The figure shows three views and two pictorial views of one solid part (mm, origin at its lowest corner). Answer the questions. A direction names the side the tool comes from. Coordinates: 2 decimals unless noted, no trailing zeros. Write each loop counter-clockwise with the first axis right and the second up, starting at its lowest first coordinate (ties: lowest second). Pieces come first, ordered by that corner, then holes.
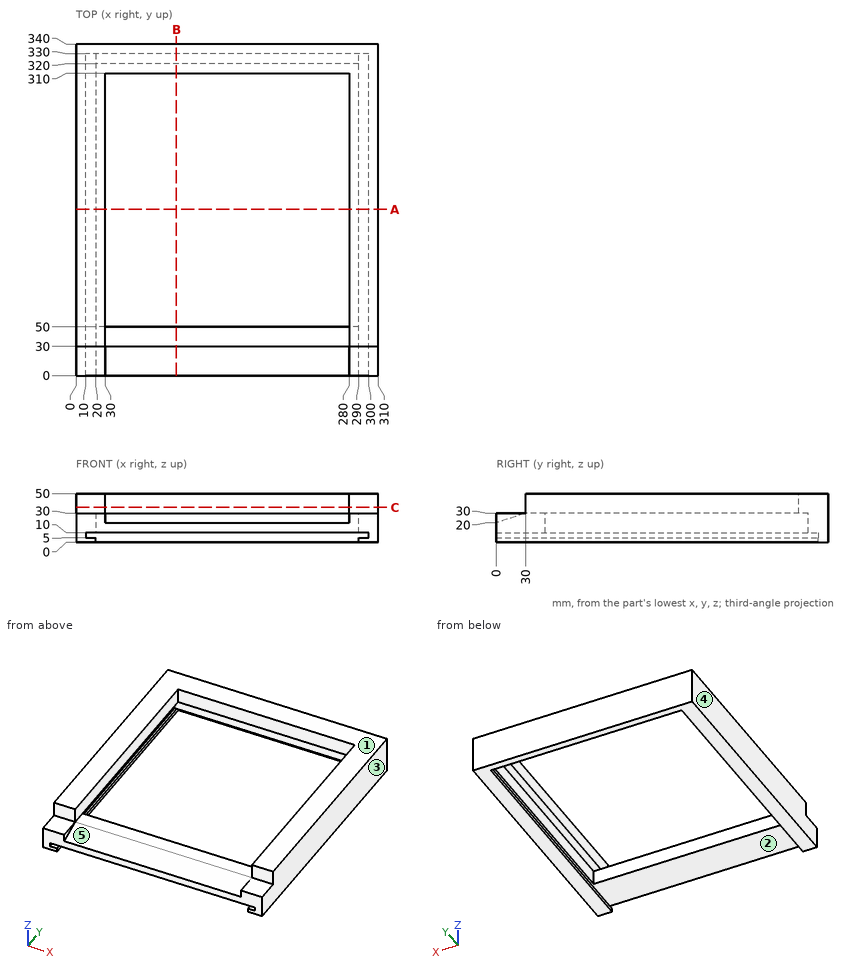
Q1. The part is cut by section B-B, the plane x = 103. Write down the section's boundary in (y, z).
Answers below:
outline: (0, 10) - (50, 10) - (50, 30) - (30, 30) - (0, 20) - close; (310, 30) - (320, 30) - (320, 10) - (330, 10) - (330, 0) - (340, 0) - (340, 50) - (310, 50) - close
Q2. Determine the mould class of the marked faces 1, 2 and 3 for opening direction X: released by +X, released by -X, zero draft, split by the parting line, or undercut.
Answers below:
face 1: zero draft
face 2: undercut
face 3: released by +X
Q3. Find the intervals of material crossed by probe 1 along X at (y, z) = (193, 42); probe 2 along Y at (x, z) = (63.5, 16.5); probe 3 along X at (y, z) = (264.5, 11.5), in increasing order.
Answers below:
probe 1: x = 0 to 30, 280 to 310
probe 2: y = 0 to 50, 320 to 340
probe 3: x = 0 to 20, 290 to 310
Q4. Given pin 1 (15 mm diameter, centred on x = 11, y = 13, fed in from +Z); pin 2 (3 mm diameter, centred on x = 82.5, z = 33, fed in from -Y); pin 3 (5 mm diameter, centred on x = 105.5, z = 2.5, fed in from -Y); pin 4 (8 mm diameter, centred on x = 250, y = 56.5, fed in from -Z), each flat-ended and moving along its own axis, determine where each tip first touches the part or whether it passes through.
Answers below:
pin 1: stops at z = 30
pin 2: stops at y = 310
pin 3: stops at y = 330
pin 4: passes through
Q5. The part is cut by section C-C, the plane z = 36. Write down the section's boundary in (x, y).
Answers below:
outline: (0, 30) - (30, 30) - (30, 310) - (280, 310) - (280, 30) - (310, 30) - (310, 340) - (0, 340) - close
Q6. The part is cut by section A-A, the plane y = 170.5. Write down the section's boundary in (x, z), then the cut area to 3 significant figures.
Answers below:
outline: (0, 0) - (20, 0) - (20, 5) - (10, 5) - (10, 10) - (20, 10) - (20, 30) - (30, 30) - (30, 50) - (0, 50) - close; (280, 30) - (290, 30) - (290, 10) - (300, 10) - (300, 5) - (290, 5) - (290, 0) - (310, 0) - (310, 50) - (280, 50) - close
area: 2,300 mm2
Q7. Which of the six approach directions +Z, -Z, +X, -X, +Y, -Y give full straight-line access (tool end or side, diameter ignored) to the marked faces 4 and 5?
Answers below:
face 4: +Z, -Z, -X, +Y, -Y
face 5: +Z, -Y
